Here's the drawing with two shaded views (mm, measured from the low corner). I have some questions. Coordinates: 2 decimals unless noted, no trailing zeros. Write each loop counter-clockwise with the first axis right and the second up, starting at its lowest first coordinate (ties: lowest second). Pieces come first, ordered by that corner, then holes.
Item 1: If we section it at D-D (z = 4.5): Please give me the cut outline in (x, y), then the cut area to 3 significant figures.
Item 2: If I drill on line 1 (Z direction, x = 1.75, y = 2.75); line 2 (Y direction, x = 2.25, z = 3.8); line 3 (Z direction, x = 0.75, y = 3.75), over which ranges is the centre line in solid material (lowest first)?
Item 3: If we section it at B-B (y = 3.5): Please give me the cut outline in (x, z).
Item 4: If we section it at C-C (z = 3.05): Please give me the cut outline in (x, y).
Item 5: If we section it at A-A (x = 3.5): Please give me the cut outline in (y, z), then the cut area to 3 significant figures.
Item 6: I'm going to push flat-ended pins straight in: pin 1 Ø3 at (y, z) = (5.5, 0.5) entering from +X; pin 2 Ø3 at (x, z) = (5.5, 4.5) entering from -Y; pin 3 Ø2.5 at (x, y) = (3.5, 3.5) entering from +Z. Where does each tip first touch, or does it pass through?
Item 7: We'd pull the mould along Y, two halves only. Please class the marked faces 1, 2 and 3: +Y half, -Y half, draft (parallel to the pull), parting line (faces both ways), or undercut.
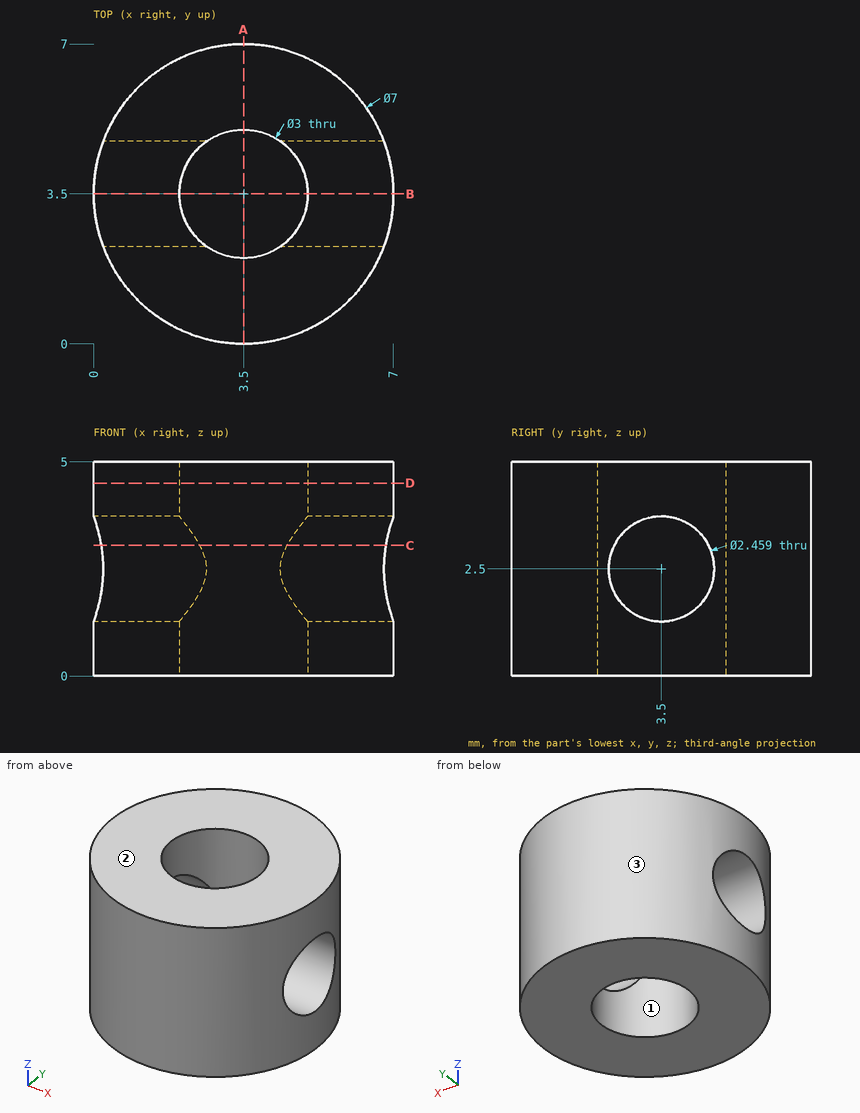
Answer list:
1. outline: circle Ø7 at (3.5, 3.5); hole circle Ø3 at (3.5, 3.5)
1. area: 31.4 mm2
2. line 1: z = 0 to 1.53, 3.47 to 5
2. line 2: y = 0.23 to 2.67, 4.33 to 6.77
2. line 3: z = 0 to 1.3, 3.7 to 5
3. outline: (0, 0) - (2, 0) - (2, 1.27) - (0, 1.27) - close; (0, 3.73) - (2, 3.73) - (2, 5) - (0, 5) - close; (5, 0) - (7, 0) - (7, 1.27) - (5, 1.27) - close; (5, 3.73) - (7, 3.73) - (7, 5) - (5, 5) - close
4. outline: (0.18, 2.4) arc R3.5 ccw to (6.82, 2.4) - (4.52, 2.4) arc R1.5 cw to (2.48, 2.4) - close; (0.18, 4.6) - (2.48, 4.6) arc R1.5 cw to (4.52, 4.6) - (6.82, 4.6) arc R3.5 ccw to start
5. outline: (0, 0) - (2, 0) - (2, 5) - (0, 5) - close; (5, 0) - (7, 0) - (7, 5) - (5, 5) - close
5. area: 20.0 mm2
6. pin 1: stops at x = 6.96
6. pin 2: stops at y = 0.04
6. pin 3: passes through
7. face 1: undercut
7. face 2: draft
7. face 3: parting line
